Work out the finished part from the listing and answer in its coordinate system (mm). A direction names the side the tool comes from. Coordinates: 2 decimals unless noted, no trailing zeros. Loops run counter-clockwise (first coordinate to the right, second up) from the corner with the lowest first, then second, coordinate; pieces in that order, holes last.
```python
from build123d import *

# Parameters (mm, degrees)
SKETCH_1_W          = 28
SKETCH_1_H          = 13.5
EXTRUDE_1_DEPTH     = 1
SKETCH_2_R          = 0.3
CUT_EXTRUDE_1_DEPTH = 32.10064308
SKETCH_2_3_W        = 5
SKETCH_2_3_H        = 6
EXTRUDE_2_DEPTH     = 1
SKETCH_2_4_R        = 0.6
CUT_EXTRUDE_2_DEPTH = 33.019525293
SKETCH_3_R          = 1
CUT_EXTRUDE_3_DEPTH = 33.019525293
SKETCH_4_W          = 7
SKETCH_4_H          = 4
CUT_EXTRUDE_4_DEPTH = 1.5
SKETCH_5_R          = 0.6
CUT_EXTRUDE_5_DEPTH = 33.019525293
SKETCH_6_W          = 1
SKETCH_6_H          = 9.5
EXTRUDE_3_DEPTH     = 1
SKETCH_7_W          = 2
SKETCH_7_H          = 6.5
SKETCH_7_R          = 0.35
SKETCH_7_H_2        = 2.5
EXTRUDE_4_DEPTH     = 1
EXTRUDE_START       = 5
SKETCH_7_3_W        = 2
SKETCH_7_3_H        = 2.5
SKETCH_7_3_R        = 0.35
SKETCH_7_3_H_2      = 6.5
EXTRUDE_5_DEPTH     = 5
SKETCH_8_W          = 0.65
SKETCH_8_H          = 9.5
EXTRUDE_6_DEPTH     = 1


with BuildPart() as part:
    # 草图1 → 凸台-拉伸1 (new body)
    with BuildSketch(Plane(origin=(0, 0, 0), x_dir=(0, 0, -1), z_dir=(1, 0, 0))):
        with Locations((-14, -6.75)):
            Rectangle(SKETCH_1_W, SKETCH_1_H)
    extrude(amount=EXTRUDE_1_DEPTH)

    # 草图2 → 切除-拉伸1 (cut, through all)
    with BuildSketch(Plane(origin=(1, 0, 0), x_dir=(0, 0, -1), z_dir=(1, 0, 0))):
        with Locations((-1.5, -4)):
            Circle(SKETCH_2_R)
        with Locations((-20.2, -2.9)):
            Circle(SKETCH_2_R)
        with Locations((-9.5, -11.6)):
            Circle(SKETCH_2_R)
    extrude(amount=-CUT_EXTRUDE_1_DEPTH, mode=Mode.SUBTRACT)

    # 草图2<3> → 凸台-拉伸2 (add)
    with BuildSketch(Plane(origin=(1, 0, 0), x_dir=(0, 0, -1), z_dir=(1, 0, 0))):
        with Locations((2.5, -12.5)):
            Rectangle(SKETCH_2_3_W, SKETCH_2_3_H)
    extrude(amount=-EXTRUDE_2_DEPTH)

    # 草图2<4> → 切除-拉伸2 (cut, through all)
    with BuildSketch(Plane(origin=(1, 0, 0), x_dir=(0, 0, -1), z_dir=(1, 0, 0))):
        with Locations((2.5, -13)):
            Circle(SKETCH_2_4_R)
    extrude(amount=-CUT_EXTRUDE_2_DEPTH, mode=Mode.SUBTRACT)

    # 草图3 → 切除-拉伸3 (cut, through all)
    with BuildSketch(Plane(origin=(1, 0, 0), x_dir=(0, 0, -1), z_dir=(1, 0, 0))):
        with Locations((-4.8, -6.15)):
            Circle(SKETCH_3_R)
        with Locations((-16.7, -6.15)):
            Circle(SKETCH_3_R)
    extrude(amount=-CUT_EXTRUDE_3_DEPTH, mode=Mode.SUBTRACT)

    # 草图4 → 切除-拉伸4 (cut)
    with BuildSketch(Plane(origin=(1, 0, 0), x_dir=(0, 0, -1), z_dir=(1, 0, 0))):
        with Locations((-26.4, -2)):
            Rectangle(SKETCH_4_W, SKETCH_4_H)
    extrude(amount=-CUT_EXTRUDE_4_DEPTH, mode=Mode.SUBTRACT)

    # 草图5 → 切除-拉伸5 (cut, through all)
    with BuildSketch(Plane.ZY):
        with Locations((22.880658046, -11.5)):
            Circle(SKETCH_5_R)
    extrude(amount=-CUT_EXTRUDE_5_DEPTH, mode=Mode.SUBTRACT)

    # 草图6 → 凸台-拉伸3 (add)
    with BuildSketch(Plane(origin=(1, 0, 0), x_dir=(0, 0, -1), z_dir=(1, 0, 0))):
        with Locations((0.5, -4.75)):
            Rectangle(SKETCH_6_W, SKETCH_6_H)
    extrude(amount=-EXTRUDE_3_DEPTH)

    # 草图7 → 凸台-拉伸4 (add)
    # profile 1 of 5: a face of its own
    with BuildSketch(Plane(origin=(1, 0, 0), x_dir=(0, 0, -1), z_dir=(1, 0, 0))):
        Polygon((-11, -13.5), (-11, -10), (-21, -10), (-21, -13.5), (-21, -20), (-11, -20), align=None)
    # profile 2 of 5: a face of its own
    with BuildSketch(Plane(origin=(1, 0, 0), x_dir=(0, 0, -1), z_dir=(1, 0, 0))):
        with Locations((-10, -16.75)):
            Rectangle(SKETCH_7_W, SKETCH_7_H)
        with Locations((-10, -19)):
            Circle(SKETCH_7_R, mode=Mode.SUBTRACT)
        with Locations((-10, -15.5)):
            Circle(SKETCH_7_R, mode=Mode.SUBTRACT)
    # profile 3 of 5: a face of its own
    with BuildSketch(Plane(origin=(1, 0, 0), x_dir=(0, 0, -1), z_dir=(1, 0, 0))):
        Polygon((-21, -20), (-21, -13.5), (-21.9, -13.5), (-21.9, -16), (-21.9, -21), (-21, -21), align=None)
    # profile 4 of 5: a face of its own
    with BuildSketch(Plane(origin=(1, 0, 0), x_dir=(0, 0, -1), z_dir=(1, 0, 0))):
        Polygon((-9, -20), (-11, -20), (-21, -20), (-21, -21), (-9, -21), align=None)
    # profile 5 of 5: a face of its own
    with BuildSketch(Plane(origin=(1, 0, 0), x_dir=(0, 0, -1), z_dir=(1, 0, 0))):
        with Locations((-22.9, -14.75)):
            Rectangle(SKETCH_7_W, SKETCH_7_H_2)
        with Locations((-22.9, -14.75)):
            Circle(SKETCH_7_R, mode=Mode.SUBTRACT)
    extrude(amount=-EXTRUDE_4_DEPTH)

    # 草图7<3> → 凸台-拉伸5 (add)
    # profile 1 of 4: a face of its own
    with BuildSketch(Plane(origin=(1, 0, 0), x_dir=(0, 0, -1), z_dir=(1, 0, 0)).offset(EXTRUDE_START)):
        Polygon((-21, -20), (-21, -13.5), (-21.9, -13.5), (-21.9, -16), (-21.9, -21), (-21, -21), align=None)
    # profile 2 of 4: a face of its own
    with BuildSketch(Plane(origin=(1, 0, 0), x_dir=(0, 0, -1), z_dir=(1, 0, 0)).offset(EXTRUDE_START)):
        with Locations((-22.9, -14.75)):
            Rectangle(SKETCH_7_3_W, SKETCH_7_3_H)
        with Locations((-22.9, -14.75)):
            Circle(SKETCH_7_3_R, mode=Mode.SUBTRACT)
    # profile 3 of 4: a face of its own
    with BuildSketch(Plane(origin=(1, 0, 0), x_dir=(0, 0, -1), z_dir=(1, 0, 0)).offset(EXTRUDE_START)):
        Polygon((-9, -20), (-9, -21), (-21, -21), (-21, -20), (-11, -20), align=None)
    # profile 4 of 4: a face of its own
    with BuildSketch(Plane(origin=(1, 0, 0), x_dir=(0, 0, -1), z_dir=(1, 0, 0)).offset(EXTRUDE_START)):
        with Locations((-10, -16.75)):
            Rectangle(SKETCH_7_3_W, SKETCH_7_3_H_2)
        with Locations((-10, -19)):
            Circle(SKETCH_7_3_R, mode=Mode.SUBTRACT)
        with Locations((-10, -15.5)):
            Circle(SKETCH_7_3_R, mode=Mode.SUBTRACT)
    extrude(amount=-EXTRUDE_5_DEPTH)

    # 草图8 → 凸台-拉伸6 (add)
    with BuildSketch(Plane(origin=(1, 0, 0), x_dir=(0, 0, -1), z_dir=(1, 0, 0))):
        with Locations((-28.325, -8.75)):
            Rectangle(SKETCH_8_W, SKETCH_8_H)
        Polygon((-28.65, -16), (-23.9, -16), (-23.9, -13.5), (-28, -13.5), (-28.65, -13.5), align=None)
    extrude(amount=-EXTRUDE_6_DEPTH)


solid = part.part
```
1. Determine the mould class of faces 1 (the flat face through (4, -13.5, 10)), 2 (the flat face through (4, -15, 23.9)), 3 (the flat face through (4, -20, 16)), 4 (the flat face through (4, -17, 21)) for opening direction Z: released by +Z, released by -Z, zero draft, split by the parting line, or undercut.
2. A cutting plane is placed at C-C, the plane x = 3.55. Give the vertices of the cut face in (y, z).
3. For faces 5 (the flat face through (0.5, -13.5, 4.6)), 6 (the flat face through (0.5, -4.8, -1)), 7 (the flat face through (4, -13.5, 22)), 8 (the flat face through (0.5, -15.5, -2.5)), determine the directions among +Z, -Z, +X, -X, +Y, -Y from which every point of the face is accessible in a straight line to the end or side of a thin tool.
4. Each of these flat-tipped pins is pushed along its axis until it touches: P1, Ø1, axis at y = -13, z = -2.5, coming from the -X side; P2, Ø3, axis at y = -5, z = 14, coming from the -X side; P3, Ø3, axis at x = 4.5, z = 22.5, coming from the +Y side; P4, Ø1.2, axis at x = 3.5, y = -14.5, coming from the +Z side. Where does it stop, or does it pass through?
5. Straight lines are drawn through the part: probe 1 along Y at (x, z) = (1.8, 10); probe 2 along Z at (x, y) = (1.4, -17); probe 3 along Y at (x, z) = (4.25, 22.9). For each, find the intervals that lie inside material, in ascending order.
6. A cutting plane is placed at D-D, the plane x = 0.65. Count the separate pieces of the cut face and the enclosed holes in it, then the cut area to 3 significant figures.
7. A cutting plane is placed at B-B, the plane y = -6.15. Give the vertices of the cut face in (x, z).
8. A cutting plane is placed at A-A, the plane z = 4.8. Give the vertices of the cut face in (x, y).
Answers below:
1. face 1: zero draft
1. face 2: released by +Z
1. face 3: undercut
1. face 4: undercut
2. outline: (-21, 9) - (-13.5, 9) - (-13.5, 11) - (-20, 11) - (-20, 21) - (-13.5, 21) - (-13.5, 23.9) - (-16, 23.9) - (-16, 21.9) - (-21, 21.9) - close; hole circle Ø0.7 at (-19, 10); hole circle Ø0.7 at (-15.5, 10); hole circle Ø0.7 at (-14.75, 22.9)
3. face 5: +X, -X, -Y
3. face 6: -Z, +X, -X, +Y
3. face 7: +Z, -Z, +X, +Y
3. face 8: -Z, +X, -X, -Y
4. P1: passes through
4. P2: stops at x = 0
4. P3: stops at y = -13.5
4. P4: stops at z = 23.9
5. probe 1: y = -21 to -19.35, -18.65 to -15.85, -15.15 to -13.5
5. probe 2: z = 9 to 11, 21 to 21.9
5. probe 3: y = -16 to -15.1, -14.4 to -13.5
6. separate pieces: 1
6. enclosed holes: 10
6. area: 506 mm2
7. outline: (0, -1) - (1, -1) - (1, 3.8) - (0, 3.8) - close; (0, 5.8) - (1, 5.8) - (1, 15.7) - (0, 15.7) - close; (0, 17.7) - (1, 17.7) - (1, 28.65) - (0, 28.65) - close
8. outline: (0, -13.5) - (1, -13.5) - (1, -7.15) - (0, -7.15) - close; (0, -5.15) - (1, -5.15) - (1, 0) - (0, 0) - close
